Geometry check sheet. Reference: the model listing, model coordinates, mm. Round coordinates to 2 decimals unless told otherwise and drop trailing zeros. Order: outer loops, then holes, each group sorted by start corner. A loop starts at its lowest first (then second) coordinate and runs counter-clockwise, first axis right, second up. Notation, with made-up numbers: (86.5, 68) - (140.5, 68) arc R29 cw to (140.5, 90) - close; hole circle Ø2 at (36, 32.25). An arc over 180 degrees is marked (long way). One line per question, with ' | ' between items. Start each with the question number.
Q1. Sectioned sample at C-C, the plane y = -136.5. Enter the section's corners in (x, z).
Q2. Material ranges on line 1 along Y through (x, z) = (197, 4.5); line 2 along Y through (x, z) = (193.5, 17); line 3 along X through (y, z) = (-326.5, 1.75), recorded low to high.
Q3. Gauge pin test, flat ends, axial feed: P1, Ø1.5, axis at y = -46.5, z = 6.5, coming from the +X side; P2, Ø2, axis at x = 286.5, z = 3.5, coming from the -Y side; P3, Ø6, axis at y = -189, z = 13.5, coming from the +X side. Record the tip position at first contact, or that the pin passes through.
Q4. Sectioned sample at B-B, the plane x = 241. Enter the section's corners in (y, z), then the cut area to 3 significant figures.
```python
from build123d import *

# Parameters (mm, degrees)
F1_DEPTH = 18


with BuildPart() as f1:
    # F0 (on Top) → F1 (new body)
    with BuildSketch(Plane.XY):
        with BuildLine():
            Line((-196.1456458643, 303.0995183934), (-556.2254190445, 303.0995183934))
            Line((-556.2254190445, 303.0995183934), (-616.1456458643, 246.8996196985))
            Line((-616.1456458643, 246.8996196985), (-616.1456458643, -391.9004816066))
            ThreePointArc((-616.1456458643, -391.9004816066), (-614.6811797702, -395.4360155125), (-611.1456458643, -396.9004816066))
            ThreePointArc((-611.1456458643, -396.9004816066), (-329.0727216352, -306.3075359847), (-147.7778268918, -71.9907044945))
            ThreePointArc((-147.7778268918, -71.9907044945), (-127.8465344688, -4.5525963575), (-117.573135126, 65.0147243663))
            ThreePointArc((-117.573135126, 65.0147243663), (-175.9949552652, 177.7420210203), (-196.1456458643, 303.0995183934))
        make_face()
        with BuildLine():
            Line((-157.8607999442, 303.0995183934), (-196.1456458643, 303.0995183934))
            ThreePointArc((-196.1456458643, 303.0995183934), (-175.9949552652, 177.7420210203), (-117.573135126, 65.0147243663))
            ThreePointArc((-117.573135126, 65.0147243663), (-116.4839005954, 84.0432775566), (-116.1206464893, 103.0995183934))
            ThreePointArc((-116.1206464893, 103.0995183934), (-126.6669028147, 205.2541076325), (-157.8607999442, 303.0995183934))
        make_face()
        with BuildLine():
            ThreePointArc((44.8805112638, -63.9526812765), (-44.8513110762, -10.1822909915), (-117.573135126, 65.0147243663))
            ThreePointArc((-117.573135126, 65.0147243663), (-127.8465344688, -4.5525963575), (-147.7778268918, -71.9907044945))
            ThreePointArc((-147.7778268918, -71.9907044945), (-52.2652669364, -48.3989008983), (44.8805112638, -63.9526812765))
        make_face()
        with BuildLine():
            Line((603.8543541357, 303.0995183934), (-157.8607999442, 303.0995183934))
            ThreePointArc((-157.8607999442, 303.0995183934), (-126.6669028147, 205.2541076325), (-116.1206464893, 103.0995183934))
            ThreePointArc((-116.1206464893, 103.0995183934), (-116.4839005954, 84.0432775566), (-117.573135126, 65.0147243663))
            ThreePointArc((-117.573135126, 65.0147243663), (-44.8513110762, -10.1822909915), (44.8805112638, -63.9526812765))
            ThreePointArc((44.8805112638, -63.9526812765), (51.9164884797, -66.7183226393), (58.8645484837, -69.6979551187))
            ThreePointArc((58.8645484837, -69.6979551187), (429.6906640365, -27.0488741975), (603.8543541357, 303.0995183934))
        make_face()
    extrude(amount=F1_DEPTH)


solid = f1.part
```
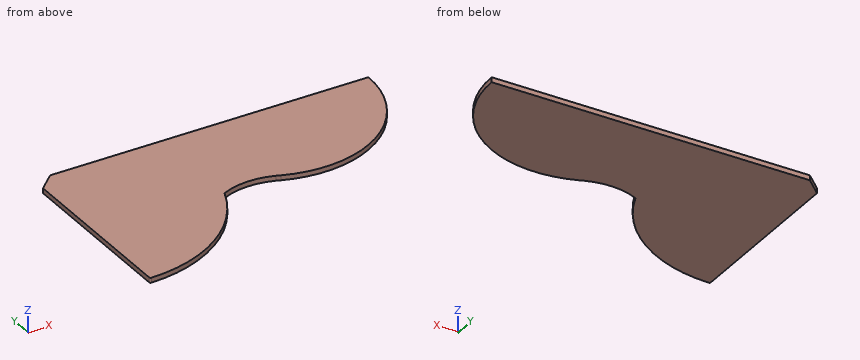
Determined:
1) outline: (-616.15, 0) - (-177.26, 0) - (-177.26, 18) - (-616.15, 18) - close
2) line 1: y = -96.84 to 303.1 | line 2: y = -96.77 to 303.1 | line 3: x = -616.15 to -360.28
3) P1: stops at x = 399.57 | P2: stops at y = -88.48 | P3: stops at x = -208.17
4) outline: (-95.17, 0) - (303.1, 0) - (303.1, 18) - (-95.17, 18) - close | area: 7,170 mm2
